Autodesk Inventor part; units mm, degrees
ref_plane "Plan de section" through (109.7586, -32.6082, 0) normal (0.2848, 0.9586, 0) x (0, 0, 1)
ref_plane "YZ Plane" through (0, 0, 0) normal (1, 0, 0) x (0, 1, 0)
ref_plane "XZ Plane" through (0, 0, 0) normal (0, 1, 0) x (-1, 0, 0)
sketch "Chemin d'esquisse" plane through (0, 0, 0) normal (0, 0, 1) x (1, 0, 0)
  arc A0 (-111.7313, 25.0274) -> (109.7586, -32.6082) centre (0, 0) ccw
  arc A1 (41.6622, 483.9245) -> (-11.2867, 473.4481) centre (17.5, 467) ccw
  arc A2 (191.7306, 243.3084) -> (186.1492, 277.6484) centre (153.387, 254.6999) ccw
  line L0 (191.7306, 243.3084) -> (109.7586, -32.6082)
  line L1 (-111.7313, 25.0274) -> (-11.2867, 473.4481)
  line L2 (41.6622, 483.9245) -> (186.1492, 277.6484)
ref_plane "Plan de section" through (109.7586, -32.6082, 0) normal (0.2848, 0.9586, 0) x (0, 0, 1)
sketch "Section" plane through (109.7586, -32.6082, 0) normal (0.2848, 0.9586, 0) x (0, 0, 1)
  line L0 (0, 2.4986) -> (0, -3.5014) construction
  line L1 (-4.25, 0) -> (4.25, 0) construction
  line L2 (-5.1594, 2.4986) -> (5.1594, 2.4986)
  line L3 (5.1594, 2.4986) -> (2.9756, -3.5014)
  line L4 (2.9756, -3.5014) -> (-2.9756, -3.5014)
  line L5 (-2.9756, -3.5014) -> (-5.1594, 2.4986)
  point P0 (0, 0)
  point P1 (0, 0)
  point P2 (0, 0)
  dimension "d0" = 8.5
  dimension "d1" = 2.4986
  dimension "d2" = 40
  dimension "d3" = 6
sweep "Courroie" add profiles "Section" path "Chemin d'esquisse"
equation "\"d0\" = da_Bw"
equation "\"d1\" = da_Hw"
equation "\"d2\" = da_Alfa"
equation "\"d3\" = da_H"
equation "\"da_Alfa\" = 40deg"
equation "\"da_H\" = 6"
equation "\"da_Bw\" = 8.5"
equation "\"da_Hw\" = 2.49859"
properties part number "Courroie trapézoïdale" material "Rubber"
Design review of the part built by this model. Coordinates are the model's own, in mm. A direction names the side the tool comes from. Round coordinates to 2 decimals unless told otherwise and drop trailing zeros. Order: outer loops, then holes, each group sorted by start corner. A loop starts at its lowest first (then second) coordinate and runs counter-clockwise, first axis right, second up. Notation, with made-up numbers: M 0,22.5 L 50,22.5 A26 ccw 50,49.5 Z; hole C 15.5,-2.5 d1. An arc over 180 degrees is marked long. Put each result on its own line as item: value.
Q1. Machinability: for faces 1 (the face through (12.8, 492.95, 3.11)), 2 (the face through (114.941, 383.664, 0.072)), 3 (the face through (112.518, 381.967, -4.083)), 4 (the face through (110.026, 380.222, -0.042)), which of the approach directions +Z, -Z, +X, -X, +Y, -Y give a long, thin tool a straight path to every point of the face, cutting with its end or side? Answer none if there is none.
Reported:
face 1: +Z
face 2: +Z, -Z, +X, +Y
face 3: -Z
face 4: +Z, -Z
Q2. Insertion check: pin 1 Ø5 at (y, z) = (199.5, -2) entering from -X. The pin has a flat end and moves straight along its axis. Give the tip position at first contact, or say it passes through.
Reported:
pin 1: x = -75.77
Q3. Consider section A-A (z = -0.5). State the section outline as (x, y) points, and give its area (3 significant figures).
Reported:
outline: M -114.17,25.57 A117 ccw 112.15,-33.32 L 194.13,242.6 A42.5 ccw 188.2,279.08 L 43.71,485.36 A32 ccw -13.72,473.99 Z; hole M -108.31,24.26 A111 ccw 106.4,-31.61 L 188.37,244.31 A36.5 ccw 183.28,275.64 L 38.79,481.92 A26 ccw -7.87,472.68 Z
area: 8,710 mm²
Q4. Consider section C-C (y = 151.5). State the section outline as (x, z) points.
Reported:
outline: M -85.96,-5.16 L -79.81,-2.98 L -79.81,2.98 L -85.96,5.16 Z; M 160.8,-2.98 L 167.06,-5.16 L 167.06,5.16 L 160.8,2.98 Z
Q5. Consider section B-B (x = 167.5). State the section outline as (y, z) points, and give its area (3 significant figures).
Reported:
outline: M 152.97,-5.16 L 174.04,-2.98 L 174.04,2.98 L 152.97,5.16 Z; M 298.17,-2.98 L 308.63,-5.16 L 308.63,5.16 L 298.17,2.98 Z
area: 256 mm²
Q6. To check wall thickness, follow line 1 (X direction, y = 449, z = 1); line 2 (X direction, y = 3, z = -2.5); line 3 (Y direction, x = 64, z = -0.5). State the ranges of each line that lie inside material, in increasing order.
Reported:
line 1: -19.32 to -13.17, 61.85 to 69.18
line 2: -116.96 to -110.96, 116.68 to 122.94
line 3: -97.94 to -90.69, 445.93 to 456.39
Q7. Draft analysis for pull direction Y (two halves, no side actions). For faces 5 (the face through (191.14, 260.59, 3.6)), 6 (the face through (153.714, 106.57, 0.072)), 7 (the face through (-64.65, 246.64, 0.07)), state which applies: released by +Y, released by -Y, zero draft, split by the parting line, or undercut.
Reported:
face 5: undercut
face 6: released by -Y
face 7: released by +Y
